Check sheet for the modelled part. Datum: model origin and axes. Units: mm. A direction names the side the tool comes from. Give positions to 0.01 mm unless a question says otherwise; leave off trailing zeros. Loops run counter-clockwise (first coordinate to the right, second up) from the corner with the lowest first, then second, coordinate; pieces in that order, holes last. Notation, with made-up numbers: (86, -4.75) -> (141, -4.75) arc R33 ccw to (141, 28.25) -> close; hole circle Ø11 at (76, 87.25). An arc over 180 degrees is marked (long way). Answer as CSV lines item,"result". Start each with the question number.
(1) Material ranges on line 1 (X direction, y = 22, z = 2); line 2 (Y direction, x = -22.5, z = 2.45); line 3 (X direction, y = 19.5, z = 1.4), recorded low to high. Write a range as from..to.
(2) Release check for a two-part mould opening along Y. For faces 5 (the face through (-19, 29, 0)), 6 (the face through (-42.37, 39.81, 1.52)), 7 (the face through (-42.421, 56.265, 1.479)), 8 (the face through (-29, 51.5, 1.5)) record: pulls with the +Y half, pulls with the -Y half, needs draft (parallel to the pull), parting line crosses it, or undercut.
(3) Gauge pin test, flat ends, axial feed: pin 1 Ø0.9 at (y, z) = (17, 1.5) entering from -X; pin 2 Ø0.9 at (x, z) = (-24, 1) entering from -Y; pin 3 Ø1 at (y, z) = (46, 2) entering from -X. Record the tip position at first contact, or that the pin passes through.
(4) Section check A-A on y = 51.5. Enter the section's corners in (x, z), plus the area to 3 significant figures.
(5) Section check B-B on x = 22.5. Enter the section's corners in (y, z), plus the area to 3 significant figures.
(6) Section check D-D on x = 5.5. Enter the section's corners in (y, z), plus the area to 3 significant figures.
(7) Section check C-C on y = 14. Enter the section's corners in (x, z).
(8) Access from +Z, -Z, +X, -X, +Y, -Y to the whole of each face (thin tool, end or side, straight path). Record for faces 1 (the face through (-11, 51, 1)), 2 (the face through (16.64, 7.4, 1.52)), 3 (the face through (-47, 28, 1)), 4 (the face through (-15.1, 7.36, 1.52)).
from build123d import *

# Parameters (mm, degrees)
SKETCH_1_W          = 55
SKETCH_1_H          = 30
SKETCH_1_R          = 1.65
EXTRUDE_1_DEPTH     = 3
SKETCH_2_W          = 55
SKETCH_2_H          = 30
EXTRUDE_2_DEPTH     = 3
EXTRUDE_3_DEPTH     = 3
SKETCH_8_R          = 1.65
CUT_EXTRUDE_1_DEPTH = 10
FILLET_2_R          = 3
CUT_EXTRUDE_2_DEPTH = 10
CUT_EXTRUDE_3_DEPTH = 92.964667128
FILLET_3_R          = 3
CUT_EXTRUDE_4_DEPTH = 88.508828254
FILLET_4_R          = 3
SKETCH_14_W         = 50
SKETCH_14_H         = 32
CUT_EXTRUDE_5_DEPTH = 88.508828254
FILLET_5_R          = 2


with BuildPart() as part:
    # 草图1 → 凸台-拉伸1 (new body)
    with BuildSketch(Plane.XY):
        with Locations((0, 11.5)):
            Rectangle(SKETCH_1_W, SKETCH_1_H)
        with Locations((-22.5, 0)):
            Circle(SKETCH_1_R, mode=Mode.SUBTRACT)
        with Locations((-22.5, 18.5)):
            Circle(SKETCH_1_R, mode=Mode.SUBTRACT)
        with Locations(Location((22.5, 18.5, 0), (0, 0, 180))):
            Circle(SKETCH_1_R, mode=Mode.SUBTRACT)
        with Locations(Location((22.5, 0, 0), (0, 0, 180))):
            Circle(SKETCH_1_R, mode=Mode.SUBTRACT)
    extrude(amount=EXTRUDE_1_DEPTH)

    # 草图2 → 凸台-拉伸2 (add)
    with BuildSketch(Plane.XY.offset(3)):
        with Locations((0, 41.5)):
            Rectangle(SKETCH_2_W, SKETCH_2_H)
    extrude(amount=-EXTRUDE_2_DEPTH)

    # 草图4 → 凸台-拉伸3 (add)
    with BuildSketch(Plane.XY.offset(3)):
        Polygon((-27.5, 26.5), (-72.5, 26.5), (-42.5, 56.5), (-27.5, 56.5), align=None)
    extrude(amount=-EXTRUDE_3_DEPTH)

    # 草图8 → 切除-拉伸1 (cut)
    with BuildSketch(Plane(origin=(0, 0, 0), x_dir=(-1, 0, 0), z_dir=(0, 0, -1))):
        with Locations((50.378679656, 44.378679656)):
            Circle(SKETCH_8_R)
    extrude(amount=-CUT_EXTRUDE_1_DEPTH, mode=Mode.SUBTRACT)

    # 圆角2
    fillet_2_edges = [part.edges().sort_by_distance(p)[0] for p in [
        (27.5, 56.5, 1.5),
        (-42.5, 56.5, 1.5),
        (27.5, -3.5, 1.5),
    ]]
    fillet(fillet_2_edges, radius=FILLET_2_R)

    # 草图9 → 切除-拉伸2 (cut)
    with BuildSketch(Plane.XY.offset(3)):
        with BuildLine():
            Line((-27.5, 53), (-17.5, 53))
            ThreePointArc((-17.5, 53), (-16, 51.5), (-17.5, 50))
            Line((-17.5, 50), (-27.5, 50))
            ThreePointArc((-27.5, 50), (-29, 51.5), (-27.5, 53))
        make_face()
    extrude(amount=-CUT_EXTRUDE_2_DEPTH, mode=Mode.SUBTRACT)

    # 草图12 → 切除-拉伸3 (cut, through all)
    with BuildSketch(Plane(origin=(0, 0, 0), x_dir=(-1, 0, 0), z_dir=(0, 0, -1))):
        Polygon((71, 28), (26, 28), (26, -3.5), (27.5, -3.5), (27.5, 26.5), (72.5, 26.5), align=None)
    extrude(amount=-CUT_EXTRUDE_3_DEPTH, mode=Mode.SUBTRACT)

    # 圆角3
    fillet_3_edges = [part.edges().sort_by_distance(p)[0] for p in [
        (-26, -3.5, 1.5),
        (-26, 28, 1.5),
        (-71, 28, 1.5),
    ]]
    fillet(fillet_3_edges, radius=FILLET_3_R)

    # 草图13 → 切除-拉伸4 (cut, through all)
    with BuildSketch(Plane(origin=(0, 0, 0), x_dir=(-1, 0, 0), z_dir=(0, 0, -1))):
        with BuildLine():
            Line((29, 38), (46.857864376, 38))
            Line((46.857864376, 38), (38.357864376, 46.5))
            Line((38.357864376, 46.5), (-17.5, 46.5))
            Line((-17.5, 46.5), (-17.5, 6.5))
            Line((-17.5, 6.5), (16, 6.5))
            Line((16, 6.5), (16, 25))
            ThreePointArc((16, 25), (19.807611845, 34.192388155), (29, 38))
        make_face()
    extrude(amount=-CUT_EXTRUDE_4_DEPTH, mode=Mode.SUBTRACT)

    # 圆角4
    fillet_4_edges = [part.edges().sort_by_distance(p)[0] for p in [
        (-16, 6.5, 1.5),
        (17.5, 6.5, 1.5),
        (17.5, 46.5, 1.5),
        (-46.857864376, 38, 1.5),
    ]]
    fillet(fillet_4_edges, radius=FILLET_4_R)

    # 草图14 → 切除-拉伸5 (cut, through all)
    with BuildSketch(Plane(origin=(0, 0, 0), x_dir=(-1, 0, 0), z_dir=(0, 0, -1))):
        with Locations((-14, 40.5)):
            Rectangle(SKETCH_14_W, SKETCH_14_H)
    extrude(amount=-CUT_EXTRUDE_5_DEPTH, mode=Mode.SUBTRACT)

    # 圆角5
    fillet_5_edges = [part.edges().sort_by_distance(p)[0] for p in [
        (-38.357864376, 46.5, 1.5),
        (-11, 46.5, 1.5),
        (17.5, 24.5, 1.5),
        (27.5, 24.5, 1.5),
        (-11, 56.5, 1.5),
    ]]
    fillet(fillet_5_edges, radius=FILLET_5_R)


solid = part.part
Working result:
1,line 1,"x = -26..-16, 17.5..27.5"
1,line 2,"y = -3.5..-1.65, 1.65..16.85, 20.15..36.26, 46.5..50, 53..56.5"
1,line 3,"x = -26..-23.81, -21.19..-16, 17.5..21.19, 23.81..27.5"
2,face 5,"needs draft"
2,face 6,"undercut"
2,face 7,"pulls with the +Y half"
2,face 8,"undercut"
3,pin 1,"stops at x = -26"
3,pin 2,"stops at y = -3.45"
3,pin 3,"stops at x = -53.5"
4,outline,"(-47.5, 0) -> (-29, 0) -> (-29, 3) -> (-47.5, 3) -> close; (-16, 0) -> (-11, 0) -> (-11, 3) -> (-16, 3) -> close"
4,area,"70.5 mm^2"
5,outline,"(-3.5, 0) -> (-1.65, 0) -> (-1.65, 3) -> (-3.5, 3) -> close; (1.65, 0) -> (16.85, 0) -> (16.85, 3) -> (1.65, 3) -> close; (20.15, 0) -> (24.5, 0) -> (24.5, 3) -> (20.15, 3) -> close"
5,area,"64.2 mm^2"
6,outline,"(-3.5, 0) -> (6.5, 0) -> (6.5, 3) -> (-3.5, 3) -> close"
6,area,"30.0 mm^2"
7,outline,"(-26, 0) -> (-16, 0) -> (-16, 3) -> (-26, 3) -> close; (17.5, 0) -> (27.5, 0) -> (27.5, 3) -> (17.5, 3) -> close"
8,face 1,"+Z, -Z, +X, +Y"
8,face 2,"+Z, -Z, +Y"
8,face 3,"+Z, -Z, -X, -Y"
8,face 4,"+Z, -Z"
